Design review of the part built by this model. Coordinates are the model's own, in mm. Face numbers are marked on the shaded views. A direction names the side the tool comes from. Round coordinates to 2 decimals unless told otherwise and drop trailing zeros. Loops run counter-clockwise (first coordinate to the right, second up) from the corner with the lowest first, then second, coordinate; pieces in that order, holes last. Notation, with made-up numbers: M 19.5,-14 L 73.5,-14 A19 ccw 73.5,3 Z; hole C 33,-13 d2. An arc over 180 degrees is marked long. Use a Markdown table: item, result.
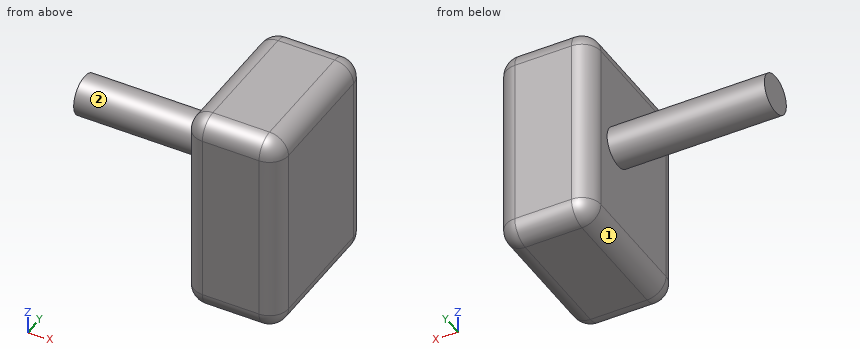
from build123d import *

# Parameters (mm, degrees)
F2_W         = 41.6020527482
F2_H         = 55.9058710933
F3_DEPTH     = 25.4
F4_R         = 5.08
F5_T1_DEPTH  = 45.7458710933
F5_T3_DEPTH  = 31.4420527482
F5_T5_DEPTH  = 15.24
F5_S9_W      = 5.08
F5_S9_H      = 5.08
F5_T10_DEPTH = 5.08
F5_S15_W     = 5.08
F5_S15_H     = 5.08
F5_T16_DEPTH = 5.08
F5_S21_W     = 5.08
F5_S21_H     = 5.08
F5_T22_DEPTH = 5.08
F5_S27_W     = 5.08
F5_S27_H     = 5.08
F5_T28_DEPTH = 5.08
F7_DEPTH     = 25.4
F8_R         = 5.2966255489
F9_DEPTH     = 67.6975995302


# Not quite as in the source:
# - a fillet or chamfer that OpenCascade refuses, or shapes differently, is made with other operations: its cross-section is extruded or revolved along the edge and cut away or added


with BuildPart() as f3:
    # F2 (on face) → F3 (new body)
    with BuildSketch(Plane.YZ):
        with Locations((20.8010263741, 27.9529355466)):
            Rectangle(F2_W, F2_H)
    extrude(amount=F3_DEPTH)

    # F4
    f4_edges = [f3.edges().sort_by_distance(p)[0] for p in [
        (12.7, 0, 0),
        (12.7, 41.602053, 0),
        (0, 20.801026, 0),
        (25.4, 20.801026, 0),
        (25.4, 41.602053, 27.952936),
        (25.4, 20.801026, 55.905871),
        (25.4, 0, 27.952936),
        (12.7, 41.602053, 55.905871),
        (0, 41.602053, 27.952936),
    ]]
    fillet(f4_edges, radius=F4_R)

    # F5: fillet of radius 5.08 on 3 edges, made by hand

    # F5_s2 → F5_t1 (cut)
    with BuildSketch(Plane.XY.offset(5.08)):
        with BuildLine():
            ThreePointArc((0, 5.08), (1.4878975516, 1.4878975516), (5.08, 0))
            Line((5.08, 0), (0, 0))
            Line((0, 0), (0, 5.08))
        make_face()
    extrude(amount=F5_T1_DEPTH, mode=Mode.SUBTRACT)

    # F5_s4 → F5_t3 (cut)
    with BuildSketch(Plane.XZ.offset(-36.5220527482)):
        with BuildLine():
            ThreePointArc((0, 50.8258710933), (1.4878975516, 54.4179735417), (5.08, 55.9058710933))
            Line((5.08, 55.9058710933), (0, 55.9058710933))
            Line((0, 55.9058710933), (0, 50.8258710933))
        make_face()
    extrude(amount=F5_T3_DEPTH, mode=Mode.SUBTRACT)

    # F5_s6 → F5_t5 (cut)
    with BuildSketch(Plane.YZ.offset(5.08)):
        with BuildLine():
            ThreePointArc((5.08, 55.9058710933), (1.4878975516, 54.4179735417), (0, 50.8258710933))
            Line((0, 50.8258710933), (0, 55.9058710933))
            Line((0, 55.9058710933), (5.08, 55.9058710933))
        make_face()
    extrude(amount=F5_T5_DEPTH, mode=Mode.SUBTRACT)


with BuildPart() as f5_tool8:
    # F5_s9 → F5_t10 (new body)
    with BuildSketch(Plane.XY.offset(50.8258710933)):
        with Locations((22.86, 2.54)):
            Rectangle(F5_S9_W, F5_S9_H)
    extrude(amount=F5_T10_DEPTH)

    # F5_s11 → F5_t12 (revolve, cut)
    with BuildSketch(Plane(origin=(20.32, 5.08, 50.8258710933), x_dir=(-0.7071067812, 0.7071067812, 0), z_dir=(0.7071067812, 0.7071067812, 0))):
        with BuildLine():
            ThreePointArc((0, -5.08), (5.08, 0), (0, 5.08))
            Line((0, 5.08), (0, -5.08))
        make_face()
    revolve(axis=Axis((20.32, 5.08, 50.8258710933), (0, 0, 1)), mode=Mode.SUBTRACT)


with BuildPart() as f3_1:
    add(f3.part)

    # F5_t7: cut F5_tool8
    add(f5_tool8.part, mode=Mode.SUBTRACT)


with BuildPart() as f5_tool14:
    # F5_s15 → F5_t16 (new body)
    with BuildSketch(Plane.YZ.offset(5.08)):
        with Locations((39.0620527482, 53.3658710933)):
            Rectangle(F5_S15_W, F5_S15_H)
    extrude(amount=-F5_T16_DEPTH)

    # F5_s17 → F5_t18 (revolve, cut)
    with BuildSketch(Plane(origin=(5.08, 36.5220527482, 50.8258710933), x_dir=(0, -0.7071067812, -0.7071067812), z_dir=(0, 0.7071067812, -0.7071067812))):
        with BuildLine():
            ThreePointArc((0, -5.08), (5.08, 0), (0, 5.08))
            Line((0, 5.08), (0, -5.08))
        make_face()
    revolve(axis=Axis((5.08, 36.5220527482, 50.8258710933), (-1, 0, 0)), mode=Mode.SUBTRACT)


with BuildPart() as f3_2:
    add(f3_1.part)

    # F5_t13: cut F5_tool14
    add(f5_tool14.part, mode=Mode.SUBTRACT)


with BuildPart() as f5_tool20:
    # F5_s21 → F5_t22 (new body)
    with BuildSketch(Plane.YZ.offset(5.08)):
        with Locations((2.54, 2.54)):
            Rectangle(F5_S21_W, F5_S21_H)
    extrude(amount=-F5_T22_DEPTH)

    # F5_s23 → F5_t24 (revolve, cut)
    with BuildSketch(Plane(origin=(5.08, 5.08, 5.08), x_dir=(0, 0.7071067812, 0.7071067812), z_dir=(0, -0.7071067812, 0.7071067812))):
        with BuildLine():
            ThreePointArc((0, -5.08), (5.08, 0), (0, 5.08))
            Line((0, 5.08), (0, -5.08))
        make_face()
    revolve(axis=Axis((5.08, 5.08, 5.08), (-1, 0, 0)), mode=Mode.SUBTRACT)


with BuildPart() as f3_3:
    add(f3_2.part)

    # F5_t19: cut F5_tool20
    add(f5_tool20.part, mode=Mode.SUBTRACT)


with BuildPart() as f5_tool26:
    # F5_s27 → F5_t28 (new body)
    with BuildSketch(Plane.YZ.offset(5.08)):
        with Locations((2.54, 53.3658710933)):
            Rectangle(F5_S27_W, F5_S27_H)
    extrude(amount=-F5_T28_DEPTH)

    # F5_s29 → F5_t30 (revolve, cut)
    with BuildSketch(Plane(origin=(5.08, 5.08, 50.8258710933), x_dir=(0, 0.7071067812, -0.7071067812), z_dir=(0, 0.7071067812, 0.7071067812))):
        with BuildLine():
            ThreePointArc((0, -5.08), (5.08, 0), (0, 5.08))
            Line((0, 5.08), (0, -5.08))
        make_face()
    revolve(axis=Axis((5.08, 5.08, 50.8258710933), (-1, 0, 0)), mode=Mode.SUBTRACT)


with BuildPart() as f3_4:
    add(f3_3.part)

    # F5_t25: cut F5_tool26
    add(f5_tool26.part, mode=Mode.SUBTRACT)

    # F6 (on face) → F7 (cut)
    with BuildSketch(Plane.YZ.offset(25.4)):
        with BuildLine():
            ThreePointArc((28.6198008208, 24.1723779255), (30.5921769571, 25.8541960079), (31.3290304018, 28.3393170685))
            ThreePointArc((31.3290304018, 28.3393170685), (28.3928704941, 32.5997711108), (23.3662914361, 31.3725764954))
            ThreePointArc((23.3662914361, 31.3725764954), (26.7699286342, 28.3393170685), (28.6198008208, 24.1723779255))
        make_face()
        with BuildLine():
            ThreePointArc((28.6198008208, 24.1723779255), (26.7699286342, 28.3393170685), (23.3662914361, 31.3725764954))
            ThreePointArc((23.3662914361, 31.3725764954), (23.0869595481, 25.652097755), (28.6198008208, 24.1723779255))
        make_face()
        with BuildLine():
            ThreePointArc((28.6198008208, 24.1723779255), (23.0869595481, 25.652097755), (23.3662914361, 31.3725764954))
            ThreePointArc((23.3662914361, 31.3725764954), (8.7034109088, 16.5279412286), (28.8466709714, 21.9696629792))
            ThreePointArc((28.8466709714, 21.9696629792), (28.7898038098, 23.0768467038), (28.6198008208, 24.1723779255))
        make_face()
    extrude(amount=F7_DEPTH, mode=Mode.SUBTRACT)

    # F8 (on face) → F9 (join)
    with BuildSketch(Plane.YZ.offset(25.4)):
        with Locations((28.2216444612, 27.5326687843)):
            Circle(F8_R)
    extrude(amount=-F9_DEPTH)


solid = f3_4.part
1. Take a section at C-C on x = -14. Give the boundary of the cut face in (y, z).
Check values:
| item | result |
|---|---|
| outline | C 28.22,27.53 d10.59 |
2. Take a section at D-D on y = 26. Give the boundary of the cut face in (x, z).
Check values:
| item | result |
|---|---|
| outline | M -42.3,22.72 L 0,22.72 L 0,5.08 A5.08 ccw 5.08,0 L 20.32,0 A5.08 ccw 25.4,5.08 L 25.4,50.83 A5.08 ccw 20.32,55.91 L 5.08,55.91 A5.08 ccw 0,50.83 L 0,32.34 L -42.3,32.34 Z |
3. Wall thickness on line 1 along X through (y, z) = (6, 16); line 2 along X through (y, z) = (25.5, 52); line 3 along Z through (x, y) = (20.5, 15.5): over which ranges is each line inside the solid? List them lowest first. Write a range as from..to.
Check values:
| item | result |
|---|---|
| line 1 | x = 0..25.4 |
| line 2 | x = 0.14..25.26 |
| line 3 | z = 0..55.9 |
4. Take a section at A-A on y = 8. Give the boundary of the cut face in (x, z).
Check values:
| item | result |
|---|---|
| outline | M 0,5.08 A5.08 ccw 5.08,0 L 20.32,0 A5.08 ccw 25.4,5.08 L 25.4,50.83 A5.08 ccw 20.32,55.91 L 5.08,55.91 A5.08 ccw 0,50.83 Z |
5. Machinability: for the marked faces 1 and 2, which of the approach directions +Z, -Z, +X, -X, +Y, -Y give a long, thin tool a straight path to every point of the face, cutting with its end or side? Answer none if there is none.
Check values:
| item | result |
|---|---|
| face 1 | -Z, -X, +Y, -Y |
| face 2 | -X |
6. Take a section at B-B on z = 20.5. Give the boundary of the cut face in (x, y).
Check values:
| item | result |
|---|---|
| outline | M 0,5.08 A5.08 ccw 5.08,0 L 20.32,0 A5.08 ccw 25.4,5.08 L 25.4,36.52 A5.08 ccw 20.32,41.6 L 5.08,41.6 A5.08 ccw 0,36.52 Z |
7. Insertion check: pin 1 (1.5 mm diameter, centred on x = -1, z = 32, fed in from -Y); pin 2 (3 mm diameter, centred on x = -26, y = 33.5, fed in from -Z); pin 3 (1 mm diameter, centred on x = 2, z = 37, fed in from -Y). Each pin has a flat end and moves straight along its axis. Give the tip position at first contact, or say it passes through.
Check values:
| item | result |
|---|---|
| pin 1 | stops at y = 24.45 |
| pin 2 | stops at z = 23.82 |
| pin 3 | stops at y = 0.7 |
